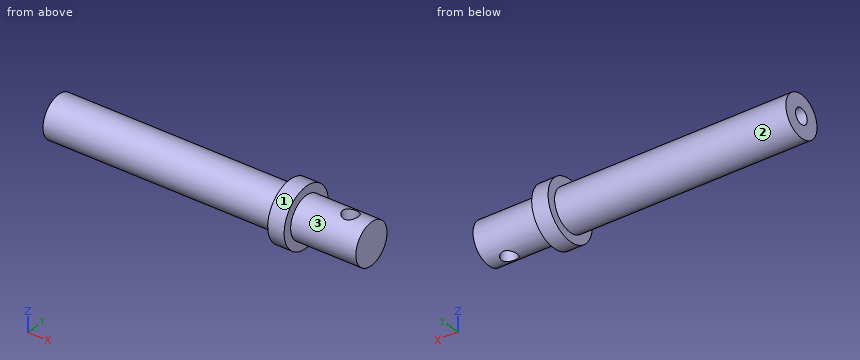
from build123d import *

# Parameters (mm, degrees)
SKETCH1_R               = 6.35
BASE_EXTRUDE_DEPTH      = 95.25
CUT_EXTRUDE1_DEPTH      = 96.672396751
CUT_EXTRUDE1_DEPTH_BACK = 96.672396751
SKETCH2_R               = 2.38125
SKETCH3_R               = 2.38125
CUT_EXTRUDE2_DEPTH      = 25.4
SKETCH4_R               = 9
EXTRUDE1_DEPTH          = 5


with BuildPart() as part:
    # Sketch1 → Base-Extrude (new body)
    with BuildSketch(Plane(origin=(0, 0, 0), x_dir=(0, 0, -1), z_dir=(1, 0, 0))):
        Circle(SKETCH1_R)
    extrude(amount=BASE_EXTRUDE_DEPTH)

    # Sketch2 → Cut-Extrude1 (cut, two sides: drawn at the far end of the back side and taken through both)
    with BuildSketch(Plane.XY.offset(-CUT_EXTRUDE1_DEPTH_BACK)):
        with Locations((88.9, 0)):
            Circle(SKETCH2_R)
    extrude(amount=CUT_EXTRUDE1_DEPTH + CUT_EXTRUDE1_DEPTH_BACK, mode=Mode.SUBTRACT)

    # Sketch3 → Cut-Extrude2 (cut)
    with BuildSketch(Plane.ZY):
        Circle(SKETCH3_R)
    extrude(amount=-CUT_EXTRUDE2_DEPTH, mode=Mode.SUBTRACT)

    # Sketch4 → Extrude1 (add)
    with BuildSketch(Plane.ZY.offset(-70.4)):
        Circle(SKETCH4_R)
    extrude(amount=-EXTRUDE1_DEPTH)


solid = part.part
Could you check a few things on this model? Use its own coordinates, in mm. Face numbers are marked on the shaded views. A direction names the side the tool comes from. Give positions to 0.01 mm unless a question says otherwise; leave off trailing zeros. Order: outer loops, then holes, each group sorted by start corner. A loop starts at its lowest first (then second) coordinate and runs counter-clockwise, first axis right, second up. Notation, with made-up numbers: (39.25, -17) - (89.25, -17) arc R21 cw to (89.25, 12) - close; hole circle Ø9 at (-29, 87.25). An arc over 180 degrees is marked (long way). One line per item, written item: value. Start each with the question number.
1. Imagine slicing it at B-B on z = 0. List the corners of the cut face in (x, y) for me, plus the area to 3 significant figures.
2. Imagine slicing it at D-D on y = 5.25. List the corners of the cut face in (x, z) for me, plus the area to 3 significant figures.
3. Imagine slicing it at C-C on x = 89. List the corners of the cut face in (y, z) for me, plus the area to 3 significant figures.
4. If I drill on probe 1 along Y at (x, z) = (18, 0); probe 2 along X at (y, z) = (0, 3); probe 3 along X at (y, z) = (7, 3.75), over which ranges is the centre line in solid material (lowest first)?
5. Imagine slicing it at A-A on y = 0. List the corners of the cut face in (x, z) for me.
6. For P1, Ø1.5, axis at x = 42.5, y = 1.5, coming from the -Z side; P2, Ø1.5, axis at y = 5.5, z = 7, coming from the -X side; P3, Ø5, axis at x = 68.5, z = 1, coming from the -Y side; P4, Ø3, axis at x = 80, z = -2, coming from the +Y side, each with a flat end and sliding along its axis, tell me the tip position at first contact or that it passes through.
7. For the marked faces 1, 2 and 3, which set-ups out of +Z, -Z, +X, -X, +Y, -Y let a thin tool reach every point of the face, with its end or its side?
Values:
1. outline: (0, -6.35) - (70.4, -6.35) - (70.4, -9) - (75.4, -9) - (75.4, -6.35) - (95.25, -6.35) - (95.25, 6.35) - (75.4, 6.35) - (75.4, 9) - (70.4, 9) - (70.4, 6.35) - (0, 6.35) - (0, 2.38) - (25.4, 2.38) - (25.4, -2.38) - (0, -2.38) - close; hole circle Ø4.76 at (88.9, 0)
1. area: 1,100 mm²
2. outline: (0, -3.57) - (70.4, -3.57) - (70.4, -7.31) - (75.4, -7.31) - (75.4, -3.57) - (95.25, -3.57) - (95.25, 3.57) - (75.4, 3.57) - (75.4, 7.31) - (70.4, 7.31) - (70.4, 3.57) - (0, 3.57) - close
2. area: 718 mm²
3. outline: (-2.38, -5.89) - (-2.38, 5.89) arc R6.35 ccw to start; (2.38, -5.89) arc R6.35 ccw to (2.38, 5.89) - close
3. area: 67.7 mm²
4. probe 1: -6.35 to -2.38, 2.38 to 6.35
4. probe 2: 0 to 86.52, 91.28 to 95.25
4. probe 3: 70.4 to 75.4
5. outline: (0, -6.35) - (70.4, -6.35) - (70.4, -9) - (75.4, -9) - (75.4, -6.35) - (86.52, -6.35) - (86.52, 6.35) - (75.4, 6.35) - (75.4, 9) - (70.4, 9) - (70.4, 6.35) - (0, 6.35) - (0, 2.38) - (25.4, 2.38) - (25.4, -2.38) - (0, -2.38) - close; (91.28, -6.35) - (95.25, -6.35) - (95.25, 6.35) - (91.28, 6.35) - close
6. P1: z = -6.31
6. P2: x = 70.4
6. P3: y = -9
6. P4: y = 6.33
7. face 1: +X, -X
7. face 2: -X
7. face 3: +X
